Read the model definition and answer for the solid it produces. Units are mm, in the model's axes. A direction names the side the tool comes from. Coordinates: 2 decimals unless noted, no trailing zeros. Order: outer loops, then holes, each group sorted by start corner. A loop starts at its lowest first (then second) coordinate and runs counter-clockwise, first axis right, second up. Notation, with made-up numbers: (-37, 39) -> (-14, 39) arc R32 cw to (-14, 76) -> close; hole circle Ø11 at (54.5, -8.5). An arc over 180 degrees is marked (long way). Return JSON: item names as keys, results as strings. Group by question number.
```python
from build123d import *

# Parameters (mm, degrees)
SKETCH2_W           = 38
SKETCH2_H           = 30
BOSS_EXTRUDE1_DEPTH = 2.032
CUT_EXTRUDE4_DEPTH  = 3.032
CUT_EXTRUDE4_TAPER  = -45
SKETCH5_R           = 1.595
CUT_EXTRUDE5_DEPTH  = 3.0320001
SKETCH6_W           = 25.7
SKETCH6_H           = 30
SKETCH6_R           = 11.75
SKETCH6_R_2         = 10.1625
BOSS_EXTRUDE4_DEPTH = 0.2874


with BuildPart() as part:
    # Sketch2 → Boss-Extrude1 (new body)
    with BuildSketch(Plane(origin=(0, 0, 0), x_dir=(1, 0, 0), z_dir=(0, 1, 0))):
        with Locations((5.811028754, 0)):
            Rectangle(SKETCH2_W, SKETCH2_H)
    extrude(amount=BOSS_EXTRUDE1_DEPTH)

    # Sketch4 → Cut-Extrude4 (cut, through all)
    with BuildSketch(Plane(origin=(0, 2.032, 0), x_dir=(1, 0, 0), z_dir=(0, 1, 0))):
        with BuildLine():
            ThreePointArc((1.5, -10), (2.207106781, -9.707106781), (2.5, -9))
            Line((2.5, -9), (2.5, 9))
            ThreePointArc((2.5, 9), (2.207106781, 9.707106781), (1.5, 10))
            Line((1.5, 10), (-1.5, 10))
            ThreePointArc((-1.5, 10), (-2.207106781, 9.707106781), (-2.5, 9))
            Line((-2.5, 9), (-2.5, -9))
            ThreePointArc((-2.5, -9), (-2.207106781, -9.707106781), (-1.5, -10))
            Line((-1.5, -10), (1.5, -10))
        make_face()
    extrude(amount=-CUT_EXTRUDE4_DEPTH, taper=CUT_EXTRUDE4_TAPER, mode=Mode.SUBTRACT)

    # Sketch5 → Cut-Extrude5 (cut, through all)
    with BuildSketch(Plane(origin=(0, 2.032, 0), x_dir=(1, 0, 0), z_dir=(0, 1, 0))):
        with Locations((18.242707696, -10)):
            Circle(SKETCH5_R)
        with Locations((18.242707696, 10)):
            Circle(SKETCH5_R)
    extrude(amount=-CUT_EXTRUDE5_DEPTH, mode=Mode.SUBTRACT)

    # Sketch6 → Boss-Extrude4 (add)
    with BuildSketch(Plane(origin=(0, 2.032, 0), x_dir=(1, 0, 0), z_dir=(0, 1, 0))):
        with Locations((-0.338971246, 0)):
            Rectangle(SKETCH6_W, SKETCH6_H)
        Circle(SKETCH6_R, mode=Mode.SUBTRACT)
        Circle(SKETCH6_R_2)
        with BuildLine():
            Line((1.5, -10), (-1.5, -10))
            ThreePointArc((-1.5, -10), (-2.207106781, -9.707106781), (-2.5, -9))
            Line((-2.5, -9), (-2.5, 9))
            ThreePointArc((-2.5, 9), (-2.207106781, 9.707106781), (-1.5, 10))
            Line((-1.5, 10), (1.5, 10))
            ThreePointArc((1.5, 10), (2.207106781, 9.707106781), (2.5, 9))
            Line((2.5, 9), (2.5, -9))
            ThreePointArc((2.5, -9), (2.207106781, -9.707106781), (1.5, -10))
        make_face(mode=Mode.SUBTRACT)
    extrude(amount=BOSS_EXTRUDE4_DEPTH)


solid = part.part
```
1. For a pull along X with two mould halves and no side action, classify faces 1 (the face through (24.811, 1, 0)), 2 (the face through (19.764, 1.03, -10.479)), 3 (the face through (-12, 2.319, 0)) as released by +X, released by -X, zero draft, split by the parting line, or undercut.
2. Straight lines are drawn through the part: L1, parallel to X at y = 2.25, z = 0; L2, parallel to Z at x = 0, y = 2.1; L3, parallel to Z at x = 17.5, y = 0.65. For each, find the intervals that lie inside material, in ascending order.
3. Find section C-C on x = 22. Determine the outline of the cut face in (y, z), and give its area (3 significant figures).
4. Which of the six approach directions +Z, -Z, +X, -X, +Y, -Y give full straight-line access (tool end or side, diameter ignored) to faces 4 (the face through (6, 1, -15)), 5 (the face through (19, 2.032, 0)), 6 (the face through (-4, 2.032, -10))?
5. Find section A-A on x = 18. Determine the outline of the cut face in (y, z), and give its area (3 significant figures).
6. Find section D-D on y = 0.8. Give the number of separate pieces and of enclosed holes in the cut face, and give its area (3 significant figures).
7. Find section B-B on z = -13. Determine the outline of the cut face in (x, y), and give its area (3 significant figures).
8. Given pin 1 (3.5 mm diameter, centred on x = 19, z = 0, fed in from +Y); pin 2 (1.9 mm diameter, centred on x = 18.24, z = -10, fed in from -Y), each flat-ended and moving along its own axis, determine where each tip first touches the part or whether it passes through.
Result:
{
 "1": {"face 1": "released by +X", "face 2": "undercut", "face 3": "zero draft"},
 "2": {"L1": "-13.19 to -11.75, -10.16 to -2.5, 2.5 to 10.16, 11.75 to 12.51", "L2": "-15 to -11.75, -10.16 to -10, 10 to 10.16, 11.75 to 15", "L3": "-15 to -11.41, -8.59 to 8.59, 11.41 to 15"},
 "3": {"outline": "(0, -15) -> (2.03, -15) -> (2.03, 15) -> (0, 15) -> close", "area": "61.0 mm^2"},
 "4": {"face 4": "-Z, +X, -X, +Y, -Y", "face 5": "+Z, -Z, +X, +Y", "face 6": "+Y"},
 "5": {"outline": "(0, -15) -> (2.03, -15) -> (2.03, -11.58) -> (0, -11.58) -> close; (0, -8.42) -> (2.03, -8.42) -> (2.03, 8.42) -> (0, 8.42) -> close; (0, 11.58) -> (2.03, 11.58) -> (2.03, 15) -> (0, 15) -> close", "area": "48.1 mm^2"},
 "6": {"separate pieces": "1", "enclosed holes": "3", "area": "961 mm^2"},
 "7": {"outline": "(-13.19, 0) -> (24.81, 0) -> (24.81, 2.03) -> (12.51, 2.03) -> (12.51, 2.32) -> (-13.19, 2.32) -> close", "area": "84.6 mm^2"},
 "8": {"pin 1": "y = 2.03", "pin 2": "through"}
}
